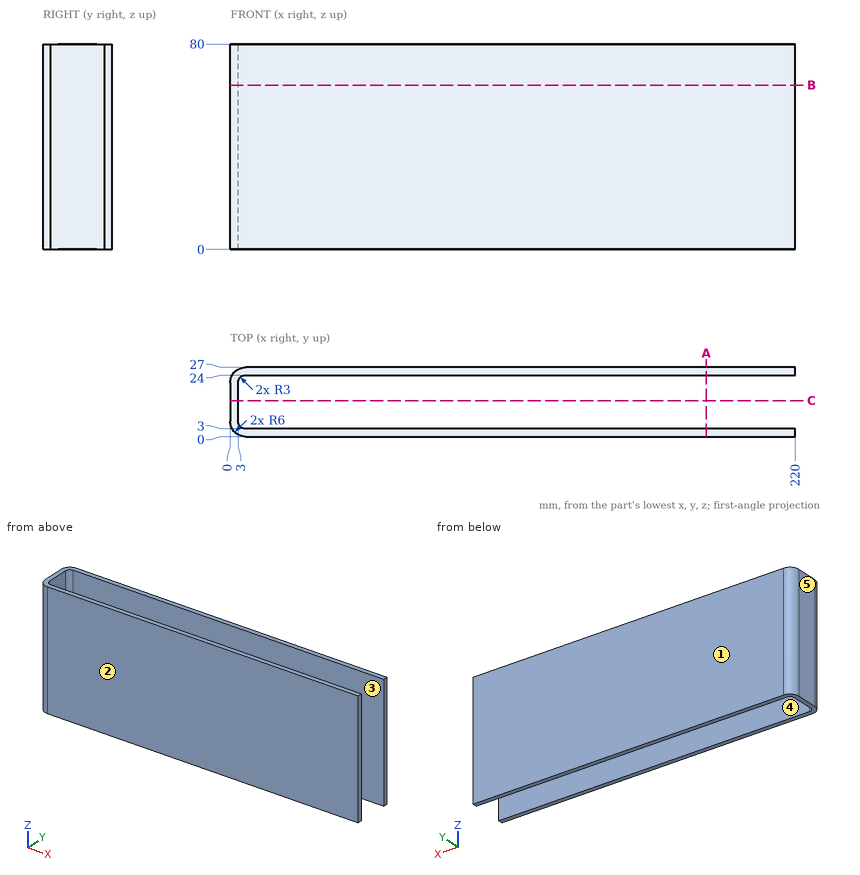
Can you work these out from the drawing? Everything is in mm from the part's minimum corner. A direction names the side the tool comes from. Give positions to 0.01 mm unless a question says otherwise; leave off trailing zeros. Write each loop counter-clockwise with the first axis right and the second up, starting at its lowest first coordinate (ties: lowest second). Pieces come first, ordered by that corner, then holes. Notation, with made-up numbers: M -5,65.5 L 13,65.5 A19 ccw 13,91.5 Z; hole C 78,15.5 d8. An arc over 180 degrees is marked long. Answer in a Markdown table with one row per item. Add a question column.
Item 1: For pin 1 Ø3 at (y, z) = (6, 70.5) entering from +X; pin 2 Ø7.5 at (y, z) = (17, 32.5) entering from +X, each with a flat end and sliding along its axis, tell me the tip position at first contact or that it passes through.
Item 2: Imagine slicing it at C-C, the plane y = 14. Write out the boundary of the cut face in (x, z).
Item 3: Imagine slicing it at B-B, the plane z = 64. Write out the boundary of the cut face in (x, y).
Item 4: Imagine slicing it at A-A, the plane x = 185.5. Write out the boundary of the cut face in (y, z), plus the area to 3 significant figures.
Item 5: Please list where these lines run through material, in increasing order: L1, parallel to Y at x = 144, z = 63; L2, parallel to X at y = 19, z = 27.5; L3, parallel to X at y = 25.75, z = 51.5.
Item 6: On a 3-axis mill with a long thin cutter (end or side, diameter ignored), from which of +Z, -Z, +X, -X, +Y, -Y can I reach the whole of each face in a straight line? I mean the marked faces 4 and 5. Say none if no direction works.
Item 7: We'd pull the mould along Y, two halves only. Please class the marked faces 1, 2 and 3: released by +Y, released by -Y, zero draft, split by the parting line, or undercut.
Evaluation:
| question | item | result |
|---|---|---|
| 1 | pin 1 | stops at x = 3.4 |
| 1 | pin 2 | stops at x = 3 |
| 2 | outline | M 0,0 L 3,0 L 3,80 L 0,80 Z |
| 3 | outline | M 0,6 A6 ccw 6,0 L 220,0 L 220,3 L 6,3 A3 cw 3,6 L 3,21 A3 cw 6,24 L 220,24 L 220,27 L 6,27 A6 ccw 0,21 Z |
| 4 | outline | M 0,0 L 3,0 L 3,80 L 0,80 Z; M 24,0 L 27,0 L 27,80 L 24,80 Z |
| 4 | area | 480 mm² |
| 5 | L1 | y = 0 to 3, 24 to 27 |
| 5 | L2 | x = 0 to 3 |
| 5 | L3 | x = 2.33 to 220 |
| 6 | face 4 | +Z, -Z, +X |
| 6 | face 5 | +Z, -Z, -X, +Y, -Y |
| 7 | face 1 | released by +Y |
| 7 | face 2 | released by -Y |
| 7 | face 3 | undercut |
